from build123d import *

# Parameters (mm, degrees)
BOSS_EXTRUDE1_DEPTH = 5.08
SKETCH2_R           = 2.032
CUT_EXTRUDE1_DEPTH  = 7.62


with BuildPart() as part:
    # Sketch1 → Boss-Extrude1 (new body)
    with BuildSketch(Plane.XY):
        Polygon((0, 0), (12.7, 0), (12.7, 7.62), (18.751410658, 7.62), (18.751410658, 13.97), (12.7, 13.97), (12.7, 39.37), (0, 39.37), (0, 13.97), (-6.051410658, 13.97), (-6.051410658, 7.62), (0, 7.62), align=None)
    extrude(amount=BOSS_EXTRUDE1_DEPTH)

    # Sketch2 → Cut-Extrude1 (cut)
    with BuildSketch(Plane.XY.offset(5.08)):
        with Locations((6.35, 30.140865425)):
            Circle(SKETCH2_R)
    extrude(amount=-CUT_EXTRUDE1_DEPTH, mode=Mode.SUBTRACT)


solid = part.part
Design review of the part built by this model. Coordinates are the model's own, in mm. A direction names the side the tool comes from. Give positions to 0.01 mm unless a question says otherwise; leave off trailing zeros. Loops run counter-clockwise (first coordinate to the right, second up) from the corner with the lowest first, then second, coordinate; pieces in that order, holes last. Notation, with made-up numbers: M 53.25,59.5 L 68.25,59.5 A27 ccw 68.25,83.5 Z; hole C 52.25,0 d2. An arc over 180 degrees is marked long. One line per question, with ' | ' between items. Start each with the question number.
1. Add section C-C (y = 21.5). Write out the cut boundary in (x, z).
2. To check wall thickness, follow L1, parallel to Y at x = 6.35, z = 3.9; L2, parallel to Y at x = 17.5, z = 0.8; L3, parallel to X at y = 17, z = 1.55. State the ranges of each line that lie inside material, in increasing order.
3. Add section B-B (z = 3.3). Write out the cut boundary in (x, y).
4. For faces 1 (the face through (12.7, 26, 3)), 2 (the face through (12.7, 4, 3)), 3 (the face through (0, 4, 3)), 4 (the face through (0, 27, 3)), list the 3-axis set-ups (+Z, -Z, +X, -X, +Y, -Y) from which the entire face can be reached by the end or side of a thin tool; tool diameter is ignored.
5. Add section D-D (x = -2). Write out the cut boundary in (y, z), plus the area to 3 significant figures.
6. Add section A-A (x = 6.35). Write out the cut boundary in (y, z).
7. Insertion check: P1, Ø1.5, axis at x = 15.5, z = 4, coming from the +Y side; P2, Ø4.5, axis at x = 6.35, y = 30.14, coming from the -Z side; P3, Ø2.5, axis at y = 30.5, z = 2.5, coming from the -X side; P4, Ø1.5, axis at y = 4, z = 1.5, coming from the +X side. Each pin has a flat end and moves straight along its axis. Give the tip position at first contact, or say it passes through.
8. The part is to be moulded in two halves that separate along Y. For faces 5 (the face through (4.74, 28.9, 2.58)), 6 (the face through (6, 39.37, 3)), 7 (the face through (6, 20, 0)), 8 (the face through (16, 7.62, 3)), say which applies: released by +Y, released by -Y, zero draft, split by the parting line, or undercut.
Worked out:
1) outline: M 0,0 L 12.7,0 L 12.7,5.08 L 0,5.08 Z
2) L1: y = 0 to 28.11, 32.17 to 39.37 | L2: y = 7.62 to 13.97 | L3: x = 0 to 12.7
3) outline: M -6.05,7.62 L 0,7.62 L 0,0 L 12.7,0 L 12.7,7.62 L 18.75,7.62 L 18.75,13.97 L 12.7,13.97 L 12.7,39.37 L 0,39.37 L 0,13.97 L -6.05,13.97 Z; hole C 6.35,30.14 d4.06
4) face 1: +Z, -Z, +X, +Y | face 2: +Z, -Z, +X, -Y | face 3: +Z, -Z, -X, -Y | face 4: +Z, -Z, -X, +Y
5) outline: M 7.62,0 L 13.97,0 L 13.97,5.08 L 7.62,5.08 Z | area: 32.3 mm²
6) outline: M 0,0 L 28.11,0 L 28.11,5.08 L 0,5.08 Z; M 32.17,0 L 39.37,0 L 39.37,5.08 L 32.17,5.08 Z
7) P1: stops at y = 13.97 | P2: stops at z = 0 | P3: stops at x = 0 | P4: stops at x = 12.7
8) face 5: undercut | face 6: released by +Y | face 7: zero draft | face 8: released by -Y
